Check sheet for the drawn part. Datum: minimum x, y, z corner. Units: mm. Round coordinates to 2 decimals unless told otherwise and drop trailing zeros. Write each loop counter-clockwise with the first axis right and the second up, starting at its lowest first coordinate (ties: lowest second). Pieces come first, ordered by that corner, then holes. Notation, with made-up numbers: M -40,63 L -9,63 A32 ccw -9,90 Z; hole C -8.75,10 d11. An arc over 180 degrees is marked long. Put each result on its own line as item: value.
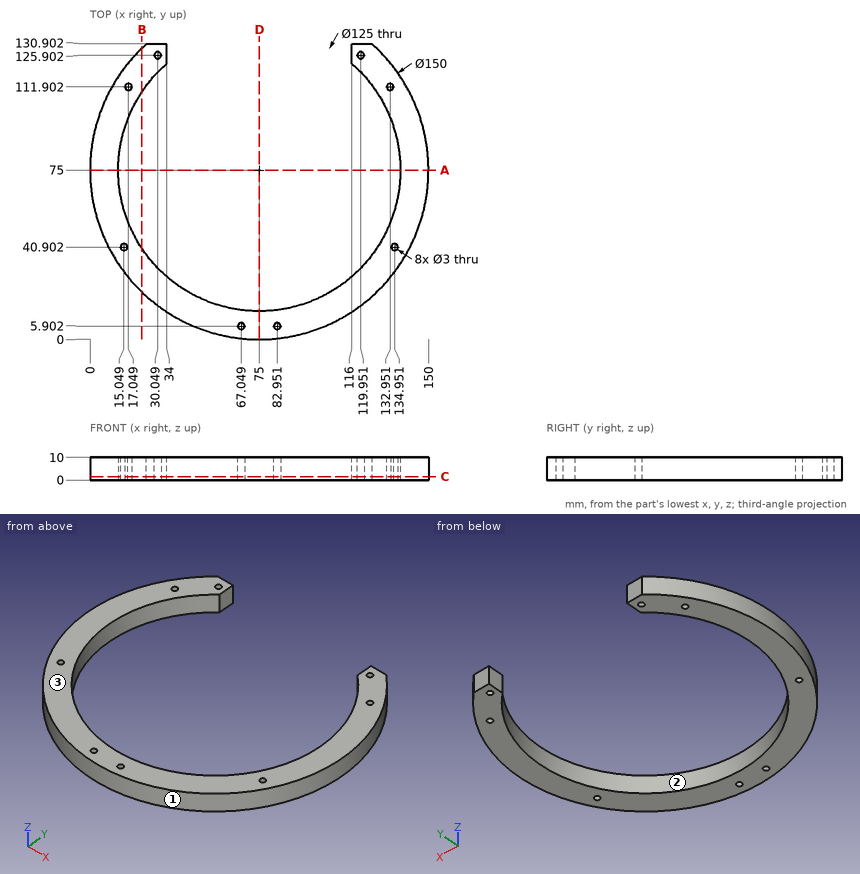
1. Cross-section at C-C (z = 1.5). Count the separate pieces of the cut face and the enclosed holes in it, then the cut area to 3 significant figures.
Computed values:
separate pieces: 1
enclosed holes: 8
area: 4,180 mm2
2. Release check for a two-part mould opening along Y. For the marked faces 1, 2 and 3 record: +Y half, -Y half, draft (parallel to the pull), parting line (faces both ways), or undercut.
Computed values:
face 1: parting line
face 2: undercut
face 3: draft
3. Cross-section at A-A (y = 75). Enter the section's corners in (x, z).
Computed values:
outline: M 0,0 L 12.5,0 L 12.5,10 L 0,10 Z; M 137.5,0 L 150,0 L 150,10 L 137.5,10 Z
4. Scan lines: probe 1 along X at (y, z) = (75, 2); probe 2 along X at (y, z) = (40.5, 2) (1 decimal); probe 3 along X at (y, z) = (30, 6) (1 decimal). Record each from-to range of solid material in increasing order.
Computed values:
probe 1: x = 0 to 12.5, 137.5 to 150
probe 2: x = 8.4 to 13.6, 16.5 to 22.9, 127.1 to 133.5, 136.4 to 141.6
probe 3: x = 15 to 31.6, 118.4 to 135
5. Depth check by flat-ended pin: pin 1 Ø1.8 at (x, y) = (119.95, 125.9) entering from -Z; pin 2 Ø4 at (x, y) = (67.05, 5.9) entering from +Z; pin 3 Ø1.5 at (y, z) = (58, 3.5) entering from -X; pin 4 Ø3 at (y, z) = (63.5, 7.5) entering from +X. Enter the tip coordinate at first touch or a pass-through.
Computed values:
pin 1: passes through
pin 2: stops at z = 10
pin 3: stops at x = 1.78
pin 4: stops at x = 149.33
6. Cross-section at B-B (x = 23). Enter the section's corners in (y, z).
Computed values:
outline: M 20.95,0 L 40.33,0 L 40.33,10 L 20.95,10 Z; M 109.67,0 L 129.05,0 L 129.05,10 L 109.67,10 Z
7. Cross-section at D-D (x = 75). Enter the section's corners in (y, z).
Computed values:
outline: M 0,0 L 12.5,0 L 12.5,10 L 0,10 Z
